from build123d import *

# Parameters (mm, degrees)
F1_DEPTH = 6
F2_W     = 4
F2_H     = 5
F3_DEPTH = 15
F4_W     = 4
F4_H     = 5
F5_DEPTH = 35


with BuildPart() as f1:
    # F0 (on Top) → F1 (new body)
    with BuildSketch(Plane.XY):
        with BuildLine():
            ThreePointArc((-15, 0), (0, 15), (15, 0))
            Line((15, 0), (15, -15))
            Line((15, -15), (20, -15))
            Line((20, -15), (20, 0))
            ThreePointArc((20, 0), (0, 20), (-20, 0))
            Line((-20, 0), (-20, -37.512027))
            Line((-20, -37.512027), (-15, -37.512027))
            Line((-15, -37.512027), (-15, 0))
        make_face()
    extrude(amount=F1_DEPTH)

    # F2 (on face) → F3 (cut)
    with BuildSketch(Plane.XZ.offset(15)):
        with Locations((17.5, 3)):
            Rectangle(F2_W, F2_H)
    extrude(amount=-F3_DEPTH, mode=Mode.SUBTRACT)

    # F4 (on face) → F5 (cut)
    with BuildSketch(Plane.XZ.offset(37.512027)):
        with Locations((-17.5, 3)):
            Rectangle(F4_W, F4_H)
    extrude(amount=-F5_DEPTH, mode=Mode.SUBTRACT)


solid = f1.part
Work out the finished part from the listing and answer in its coordinate system (mm). A direction names the side the tool comes from. Coordinates: 2 decimals unless noted, no trailing zeros. Loops run counter-clockwise (first coordinate to the right, second up) from the corner with the lowest first, then second, coordinate; pieces in that order, holes last. Notation, with made-up numbers: M 29,-13 L 40,-13 A28 cw 40,21 Z; hole C -39.75,-21.75 d10. An arc over 180 degrees is marked long. Answer in a Markdown table with one row per item. Add a question column.
1. Consider L1, parallel to X at y = -10, z = 3.1; L2, parallel to X at y = -32, z = 2.05; L3, parallel to Z at x = -18, y = -15.5. Determine where each line is inside the solid, lowest interval first.
2. Find section D-D, the plane x = 0. Write down the section's boundary in (y, z), then the cut area to 3 significant figures.
3. Find section B-B, the plane y = 1. Write down the section's boundary in (x, z), then the cut area to 3 significant figures.
4. A tool of negligible diameter and unlimited length cuts with its end or side. For faces 5 (the flat face through (-20, -18, 3)), 6 (the flat face through (-15.5, -20, 3)), 7 (the flat face through (15.2, -15, 3)), 8 (the flat face through (15, -7, 3)), 9 (the flat face through (-19.8, -37.512, 3)), from which of +Z, -Z, +X, -X, +Y, -Y can it reach the whole face along a straight path? Write none if from no direction.
5. Find section A-A, the plane y = -31. Write down the section's boundary in (x, z), then the cut area to 3 significant figures.
6. Flat-ended cylindrical pins translate along their axes: P1, Ø3, axis at x = 11.5, z = 3.5, coming from the -Y side; P2, Ø1.2, axis at x = -16.5, y = -24, coming from the -Z side; P3, Ø3, axis at x = -8, z = 1.5, coming from the +Y side; P4, Ø1.8, axis at y = -17.5, z = 4, coming from the +X side. Find the tip coordinate at first contact, or state that the pin passes through.
7. The mould has two halves that part along X. Classify faces 1 (the flat face through (17, -8, 5.5)), 2 (the flat face through (15.5, -8, 3)), 3 (the flat face through (-15, 4, 0)), 4 (the cylindrical face through (0, 20, 3)): pulls with the +X half, pulls with the -X half, needs draft (parallel to the pull), parting line crosses it, or undercut.
8. Find section C-C, the plane z = 2.2. Write down the section's boundary in (x, y).
Reported:
| question | item | result |
|---|---|---|
| 1 | L1 | x = -20 to -19.5, -15.5 to -15, 15 to 15.5, 19.5 to 20 |
| 1 | L2 | x = -20 to -19.5, -15.5 to -15 |
| 1 | L3 | z = 0 to 0.5, 5.5 to 6 |
| 2 | outline | M 15,0 L 20,0 L 20,6 L 15,6 Z |
| 2 | area | 30.0 mm^2 |
| 3 | outline | M -19.97,0 L -14.97,0 L -14.97,6 L -19.97,6 Z; M 14.97,0 L 19.97,0 L 19.97,6 L 14.97,6 Z |
| 3 | area | 60.1 mm^2 |
| 4 | face 5 | +Z, -Z, -X, +Y, -Y |
| 4 | face 6 | -Y |
| 4 | face 7 | +Z, -Z, +X, -Y |
| 4 | face 8 | +Z, -Z, -Y |
| 4 | face 9 | +Z, -Z, +X, -X, -Y |
| 5 | outline | M -20,0 L -15,0 L -15,6 L -20,6 Z; hole M -19.5,0.5 L -15.5,0.5 L -15.5,5.5 L -19.5,5.5 Z |
| 5 | area | 10.0 mm^2 |
| 6 | P1 | stops at y = 7.48 |
| 6 | P2 | stops at z = 0 |
| 6 | P3 | stops at y = 18.91 |
| 6 | P4 | stops at x = -15 |
| 7 | face 1 | undercut |
| 7 | face 2 | undercut |
| 7 | face 3 | needs draft |
| 7 | face 4 | parting line crosses it |
| 8 | outline | M -20,-37.51 L -19.5,-37.51 L -19.5,-2.51 L -15.5,-2.51 L -15.5,-37.51 L -15,-37.51 L -15,0 A15 cw 15,0 L 15,-15 L 15.5,-15 L 15.5,0 L 19.5,0 L 19.5,-15 L 20,-15 L 20,0 A20 ccw -20,0 Z |
